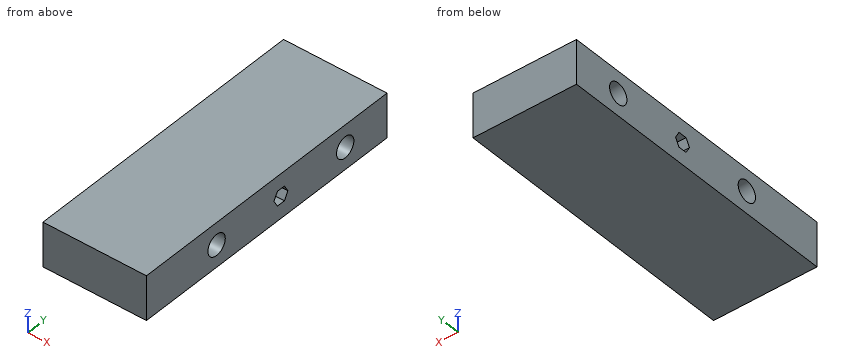
Autodesk Inventor part; units mm, degrees
ref_plane "YZ Plane" through (0, 0, 0) normal (1, 0, 0) x (0, 1, 0)
ref_plane "XZ Plane" through (0, 0, 0) normal (0, 1, 0) x (-1, 0, 0)
ref_plane "XY Plane" through (0, 0, 0) normal (0, 0, 1) x (1, 0, 0)
sketch "Sketch4" plane through (0, 0, 0) normal (0, 1, 0) x (-1, 0, 0)
  line L0 (44.45, 19.05) -> (-44.45, 19.05)
  line L1 (-44.45, 19.05) -> (-44.45, -19.05)
  line L2 (-44.45, -19.05) -> (44.45, -19.05)
  line L3 (44.45, -19.05) -> (44.45, 19.05)
  line L4 (44.45, 19.05) -> (-44.45, -19.05) construction
  line L5 (-44.45, 19.05) -> (44.45, -19.05) construction
  point P0 (0, 0)
  dimension "d8" = 88.9
  dimension "d9" = 38.1
extrude "Extrusion2" add sketch "Sketch4" along normal mid plane 250
sketch "Sketch5" plane through (44.45, -125, -19.05) normal (1, 0, 0) x (0, 0, -1)
  circle A0 centre (-19.05, 206.558) radius 9
  circle A1 centre (-19.05, 72.932) radius 9
  line L0 (-38.1, 250) -> (0, 250)
  circle A2 centre (-19.05, 139.745) radius 7.2555
  line L1 (-19.05, 132.4895) -> (-25.3334, 136.1172)
  line L2 (-25.3334, 136.1172) -> (-25.3334, 143.3727)
  line L3 (-25.3334, 143.3727) -> (-19.05, 147.0005)
  line L4 (-19.05, 147.0005) -> (-12.7666, 143.3727)
  line L5 (-12.7666, 143.3727) -> (-12.7666, 136.1173)
  line L6 (-12.7666, 136.1173) -> (-19.05, 132.4895)
  point P0 (-19.05, 125)
  dimension "d40" = 14.511
  dimension "d12" = 18
  dimension "d14" = 18
  dimension "d37" = 43.442
  dimension "d38" = 66.813
  dimension "d39" = 133.626
  dimension "d41" = 66.813
extrude "Extrusion4" cut sketch "Sketch5" against normal blind 103.1875 contours A0 | A1 | L5 L6 L1 L2 L3 L4
properties part number "CNC-Y-axis- moving side to side plateform"
Can you work these out from the model? Positions are in its coordinate system, mm. Round coordinates to 2 decimals unless told otherwise and drop trailing zeros. Order: outer loops, then holes, each group sorted by start corner. A loop starts at its lowest first (then second) coordinate and runs counter-clockwise, first axis right, second up. Notation, with made-up numbers: (24.5, 10) -> (33.5, 10) arc R17 cw to (33.5, 36) -> close; hole circle Ø6 at (75, 7). An arc over 180 degrees is marked (long way). Write each question's results on one line, items separated by ' | '. Start each with the question number.
Item 1: If we section it at A-A, the plane y = 84: Write out the boundary of the cut face in (x, z), then the cut area to 3 significant figures.
Item 2: Please list where these lines run through material, in increasing order: L1, parallel to Y at x = -11.5, z = 0; L2, parallel to Y at x = 5, z = -3; L3, parallel to Y at x = -19.5, z = 6.5.
Item 3: If we section it at B-B, the plane x = -27: Write out the boundary of the cut face in (y, z), then the cut area to 3 significant figures.
Results:
1) outline: (-44.45, -19.05) -> (44.45, -19.05) -> (44.45, -8.66) -> (-44.45, -8.66) -> close; (-44.45, 8.66) -> (44.45, 8.66) -> (44.45, 19.05) -> (-44.45, 19.05) -> close | area: 1,850 mm2
2) L1: y = -125 to -61.07, -43.07 to 7.49, 22 to 72.56, 90.56 to 125 | L2: y = -125 to -60.55, -43.58 to 9.22, 20.27 to 73.07, 90.04 to 125 | L3: y = -125 to -58.29, -45.84 to 75.33, 87.78 to 125
3) outline: (-125, -19.05) -> (125, -19.05) -> (125, 19.05) -> (-125, 19.05) -> close; hole circle Ø18 at (-52.07, 0); hole (7.49, 0) -> (11.12, -6.28) -> (18.37, -6.28) -> (22, 0) -> (18.37, 6.28) -> (11.12, 6.28) -> close; hole circle Ø18 at (81.56, 0) | area: 8,880 mm2
